The listing builds one solid part. Answer for the finished solid, in the listing's coordinates (mm). Face numbers are marked on the shaded views. A direction names the side the tool comes from. Coordinates: 2 decimals unless noted, no trailing zeros. Order: outer loops, then holes, each group sorted by start corner. A loop starts at its lowest first (then second) coordinate and runs counter-clockwise, first axis right, second up. Notation, with made-up numbers: M 74,78 L 129,78 A9 ccw 129,87 Z; hole C 16.25,62 d3. An arc over 180 degrees is marked long. One line per item, written item: value. Start each with the question number.
Q1. Determine the mould class of the marked faces 4, 5, 6 and 7 for opening direction Z: pulls with the +Z half, pulls with the -Z half, needs draft (parallel to the pull), parting line crosses it, or undercut.
Q2. For the marked faces 1, 2 and 3, determine the directions among +Z, -Z, +X, -X, +Y, -Y from which every point of the face is accessible in a straight line to the end or side of a thin tool.
Q3. Each of these flat-tipped pins is pushed along its axis until it touches: pin 1 Ø1.5 at (x, y) = (-6, 8) entering from -Z; pin 2 Ø1.5 at (y, z) = (2, 30) entering from -X; pin 3 Ø9 at (x, y) = (5, -1) entering from +Z; pin 4 Ø1 at (x, z) = (6, 27) entering from -Y. Where does it stop, or does it pass through?
Q4. The part is cut by section A-A on y = 8.5. Give the vertices of the cut face in (x, z), then the cut area to 3 significant figures.
Q5. Straight lines are drawn through the part: line 1 along Z through (x, y) = (-3.75, 1); line 2 along Z through (x, y) = (4, 1.75); line 3 along Z through (x, y) = (-6.5, -1.5). For each, find the intervals that lie inside material, in ascending order. Write a range as [from, to].
Autodesk Inventor part; units mm, degrees
ref_plane "YZ Plane" through (0, 0, 0) normal (1, 0, 0) x (0, 1, 0)
ref_plane "XZ Plane" through (0, 0, 0) normal (0, 1, 0) x (-1, 0, 0)
ref_plane "XY Plane" through (0, 0, 0) normal (0, 0, 1) x (1, 0, 0)
sketch "Sketch1" plane through (0, 0, 0) normal (0, 0, 1) x (1, 0, 0)
  line L0 (-3.4267, 10.372) -> (10.6957, -2.2184)
  line L1 (10.6957, -2.2184) -> (-7.2691, -8.1536)
  line L2 (-7.2691, -8.1536) -> (-3.4267, 10.372)
  ellipse E0 centre (0, 0) end of major axis (3.175, 0) minor radius 2.667
  dimension "d1" = 3.175
  dimension "d2" = 2.667
  dimension "d0" = 14.1224
extrude "Extrusion1" add sketch "Sketch1" along normal blind 8.128 contours L0 L1 L2 | E0
ref_plane "Work Plane2" through (0, 0, 12.954) normal (0, 0, 1) x (1, 0, 0)
sketch "Sketch2" plane through (0, 0, 12.954) normal (0, 0, 1) x (1, 0, 0)
  point P0 (0, 0)
sketch "Sketch3" plane through (0, 0, 12.954) normal (0, 0, 1) x (1, 0, 0)
  point P0 (0, 0)
sketch "Sketch4" plane through (0, 0, 12.954) normal (0, 0, 1) x (1, 0, 0)
  ellipse E0 centre (0, 0) end of major axis (3.175, 0) minor radius 2.667
  dimension "d6" = 3.175
  dimension "d7" = 2.667
sketch "Sketch5" plane through (0, 0, 12.954) normal (0, 0, 1) x (1, 0, 0)
  line L0 (10.6957, -2.2184) -> (-3.4267, 10.372)
  line L1 (-3.4267, 10.372) -> (-7.2691, -8.1536)
  line L2 (-7.2691, -8.1536) -> (10.6957, -2.2184)
sketch "Sketch6" plane through (0, 0, 8.128) normal (0, 0, 1) x (1, 0, 0)
  ellipse E0 centre (0, 0) end of major axis (3.175, 0) minor radius 2.667
  ellipse E1 centre (0, 0) end of major axis (3.175, 0) minor radius 2.667
loft "Loft1" add profiles "Sketch6", "Sketch4"
ref_plane "Work Plane4" through (0, 0, 30.734) normal (0, 0, 1) x (1, 0, 0)
ref_plane "Work Plane3" through (0, 0, 22.098) normal (0, 0, 1) x (1, 0, 0)
sketch "Sketch7" plane through (0, 0, 22.098) normal (0, 0, 1) x (1, 0, 0)
  ellipse E0 centre (0, 0) end of major axis (-3.175, 0) minor radius 2.667
sketch "Sketch8" plane through (0, 0, 22.098) normal (0, 0, 1) x (1, 0, 0)
  ellipse E0 centre (0, 0) end of major axis (3.175, 0) minor radius 2.667
  ellipse E1 centre (0, 0) end of major axis (-3.175, 0) minor radius 2.667
sketch "Sketch9" plane through (0, 0, 12.954) normal (0, 0, 1) x (1, 0, 0)
  ellipse E0 centre (0, 0) end of major axis (7.62, 0) minor radius 5.08
  dimension "d16" = 7.62
  dimension "d17" = 5.08
loft "Loft2" add profiles "Sketch9", "Sketch7"
sketch "Sketch10" plane through (0, 0, 30.734) normal (0, 0, 1) x (1, 0, 0)
  ellipse E0 centre (0, 0) end of major axis (9.144, 0) minor radius 6.858
  dimension "d22" = 6.858
  dimension "d23" = 9.144
loft "Loft3" add profiles "Sketch10" section 1 edges at (0, 2.667, 22.098) (0, -2.667, 22.098)
sketch "Sketch11" plane through (0, 0, 30.734) normal (0, 0, 1) x (1, 0, 0)
  line L0 (-3.175, 3.175) -> (3.175, 3.175)
  line L1 (3.175, 3.175) -> (3.175, -3.175)
  line L2 (3.175, -3.175) -> (-3.175, -3.175)
  line L3 (-3.175, -3.175) -> (-3.175, 3.175)
  point P0 (0, 0)
  dimension "d28" = 6.35
  dimension "d29" = 6.35
  dimension "d30" = 3.175
  dimension "d31" = 3.175
extrude "Extrusion2" add sketch "Sketch11" along normal blind 6.35
fillet "Fillet1" radius 3.175 1 edges at (3.175, 0, 37.084)
fillet "Fillet2" radius 3.175 1 edges at (-3.175, 0, 37.084)
fillet "Fillet3" radius 3.175 3 edges at (3.175, 3.175, 32.3215) (2.2451, 3.175, 36.1541) (-3.175, 3.175, 32.3215)
fillet "Fillet4" radius 3.175 3 edges at (3.175, -3.175, 32.3215) (2.2451, -3.175, 36.1541) (-3.175, -3.175, 32.3215)
properties part number "girlNT"
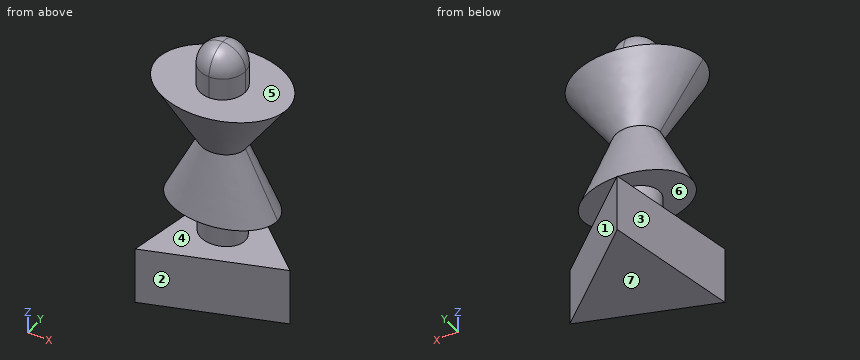
Output:
1. face 4: undercut
1. face 5: pulls with the +Z half
1. face 6: undercut
1. face 7: pulls with the -Z half
2. face 1: -Z, +X, +Y
2. face 2: -Z, +X, -Y
2. face 3: -Z, -X, +Y
3. pin 1: passes through
3. pin 2: stops at x = -8.83
3. pin 3: stops at z = 37.03
3. pin 4: stops at y = -2.92
4. outline: M -3.81,0 L -1.33,0 L -1.33,8.13 L -3.81,8.13 Z
4. area: 20.2 mm^2
5. line 1: z = [0, 8.13], [12.95, 20.48], [23.21, 30.73]
5. line 2: z = [0, 8.13], [12.95, 19.09], [24.1, 30.73]
5. line 3: z = [12.95, 14.51], [27.33, 30.73]
